```python
from build123d import *

# Parameters (mm, degrees)
SKETCH_W     = 30
SKETCH_H     = 66.5
SKETCH_R     = 1.6
PAD_DEPTH    = 8.5
SKETCH001_R  = 4
POCKET_DEPTH = 5
FILLET_R     = 1


with BuildPart() as part:
    # Sketch → Pad (new body)
    with BuildSketch(Plane.XY):
        with Locations((15, 33.25)):
            Rectangle(SKETCH_W, SKETCH_H)
        with Locations((7.5, 40)):
            Circle(SKETCH_R, mode=Mode.SUBTRACT)
        with Locations((22.5, 40)):
            Circle(SKETCH_R, mode=Mode.SUBTRACT)
    extrude(amount=PAD_DEPTH)

    # Sketch001 (on Face8 of Pad) → Pocket (cut)
    with BuildSketch(Plane.XY.offset(8.5)):
        with Locations((7.5, 40)):
            Circle(SKETCH001_R)
        with Locations((22.5, 40)):
            Circle(SKETCH001_R)
    extrude(amount=-POCKET_DEPTH, mode=Mode.SUBTRACT)

    # Fillet
    fillet_edges = [part.edges().sort_by_distance(p)[0] for p in [
        (15, 66.5, 8.5),
        (15, 0, 8.5),
    ]]
    fillet(fillet_edges, radius=FILLET_R)


solid = part.part
```
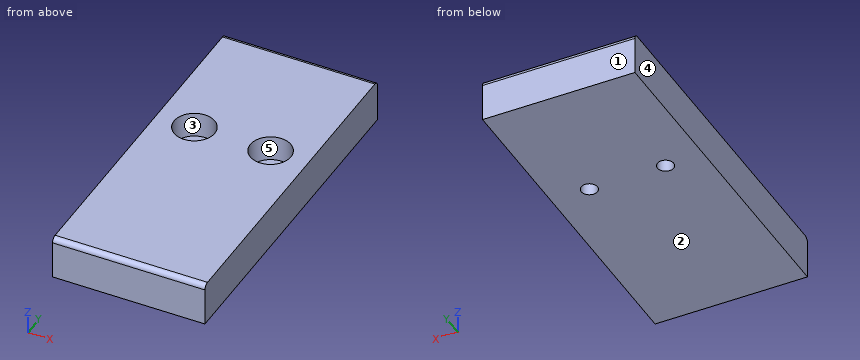
Source: CAD feature listing. Evaluate the final solid. Frame: model axes, mm. Face numbers are marked on the shaded views. A direction names the side the tool comes from. Round coordinates to 2 decimals unless told otherwise and drop trailing zeros. Loops run counter-clockwise (first coordinate to the right, second up) from the corner with the lowest first, then second, coordinate; pieces in that order, holes last. Notation, with made-up numbers: (-14, 38.5) - (37, 38.5) arc R27 ccw to (37, 71.5) - close; hole circle Ø1 at (77.25, 89.5). An arc over 180 degrees is marked (long way). Use CSV: the item, a comma, the result in double quotes.
Q1. Reachability of the marked faces 4 and 5 from +Z, -Z, +X, -X, +Y, -Y: full face, straight path, thin tool, end or side. Return the list, or none.
Reported:
face 4,"+Z, -Z, -X, +Y, -Y"
face 5,"+Z"
Q2. Section query A-A, the plane x = 22.5. Output: boundary loops of the cut face in (y, z).
Reported:
outline,"(0, 0) - (38.4, 0) - (38.4, 3.5) - (36, 3.5) - (36, 8.5) - (1, 8.5) arc R1 ccw to (0, 7.5) - close; (41.6, 0) - (66.5, 0) - (66.5, 7.5) arc R1 ccw to (65.5, 8.5) - (44, 8.5) - (44, 3.5) - (41.6, 3.5) - close"
Q3. Section query C-C, the plane z = 6.5. Output: boundary loops of the cut face in (x, y).
Reported:
outline,"(0, 0) - (30, 0) - (30, 66.5) - (0, 66.5) - close; hole circle Ø8 at (7.5, 40); hole circle Ø8 at (22.5, 40)"
Q4. Section query D-D, the plane x = 5.25. Output: boundary loops of the cut face in (y, z), then the cut area to 3 significant figures.
Reported:
outline,"(0, 0) - (66.5, 0) - (66.5, 7.5) arc R1 ccw to (65.5, 8.5) - (43.31, 8.5) - (43.31, 3.5) - (36.69, 3.5) - (36.69, 8.5) - (1, 8.5) arc R1 ccw to (0, 7.5) - close"
area,"532 mm^2"
Q5. Ray query, line 1 along X through (y, z) = (40, 1.65); line 2 along Y through (x, z) = (7.5, 5.65); line 3 along Y through (x, z) = (7.5, 0.8). Return the intervals inside material, ascending.
Reported:
line 1,"0 to 5.9, 9.1 to 20.9, 24.1 to 30"
line 2,"0 to 36, 44 to 66.5"
line 3,"0 to 38.4, 41.6 to 66.5"
Q6. Section query B-B, the plane y = 40. Output: boundary loops of the cut face in (x, z), then the cut area to 3 significant figures.
Reported:
outline,"(0, 0) - (5.9, 0) - (5.9, 3.5) - (3.5, 3.5) - (3.5, 8.5) - (0, 8.5) - close; (9.1, 0) - (20.9, 0) - (20.9, 3.5) - (18.5, 3.5) - (18.5, 8.5) - (11.5, 8.5) - (11.5, 3.5) - (9.1, 3.5) - close; (24.1, 0) - (30, 0) - (30, 8.5) - (26.5, 8.5) - (26.5, 3.5) - (24.1, 3.5) - close"
area,"153 mm^2"
Q7. Pin query (flat end, axial travel): pin 1 Ø2 at (x, y) = (22.5, 49) entering from -Z; pin 2 Ø5 at (x, y) = (7.5, 40) entering from +Z. Return the tip coordinate at first contact, or that it passes through.
Reported:
pin 1,"z = 0"
pin 2,"z = 3.5"
Q8. Mould query, pull axis Y, two halves, no side actions, for the marked faces 1, 2 and 3. Classes: pulls with the +Y half, pulls with the -Y half, needs draft (parallel to the pull), parting line crosses it, or undercut.
Reported:
face 1,"pulls with the +Y half"
face 2,"needs draft"
face 3,"undercut"
